```python
from build123d import *

# Parameters (mm, degrees)
EXTRUDE1_DEPTH     = 12.7
SKETCH4_R          = 6.35
CUT_EXTRUDE1_DEPTH = 13.7
CHAMFER2_SIZE      = 0.762


with BuildPart() as part:
    # Sketch2 → Extrude1 (new body)
    with BuildSketch(Plane.XY):
        Polygon((8.798818102, 0), (4.399409051, 7.62), (-4.399409051, 7.62), (-8.798818102, 0), (-4.399409051, -7.62), (4.399409051, -7.62), align=None)
    extrude(amount=EXTRUDE1_DEPTH)

    # Sketch4 → Cut-Extrude1 (cut, through all)
    with BuildSketch(Plane.XY.offset(12.7)):
        Circle(SKETCH4_R)
    extrude(amount=-CUT_EXTRUDE1_DEPTH, mode=Mode.SUBTRACT)

    # Chamfer2
    chamfer2_edges = [part.edges().sort_by_distance(p)[0] for p in [
        (0, 7.62, 12.7),
        (-6.599113577, 3.81, 12.7),
        (-6.599113577, -3.81, 12.7),
        (0, -7.62, 12.7),
        (6.599113577, -3.81, 12.7),
        (6.599113577, 3.81, 12.7),
    ]]
    chamfer(chamfer2_edges, length=CHAMFER2_SIZE)


solid = part.part
```
Check sheet for the modelled part. Datum: model origin and axes. Units: mm. Give positions to 0.01 mm unless a question says otherwise; leave off trailing zeros. Write each loop counter-clockwise with the first axis right and the second up, starting at its lowest first coordinate (ties: lowest second). Pieces come first, ordered by that corner, then holes. Notation, with made-up numbers: (33, 25.5) - (91, 25.5) arc R22 ccw to (91, 64.5) - close; hole circle Ø6 at (82.5, 38). An arc over 180 degrees is marked (long way). Answer as a JSON object with one key per item and string values. Group by question number.
1) Sectioned sample at A-A (x = 0). Record the cut outline in (y, z).
2) Thickness scan on probe 1 along Y at (x, z) = (0, 4.75); probe 2 along Y at (x, z) = (-1.75, 4.5); probe 3 along X at (y, z) = (3.75, 8.5). Record the ranges inside material, lowest first. Write a range as from..to.
3) Release check for a two-part mould opening along X. For faces 1 (the face through (-1.38, -6.2, 6.44)), 2 (the face through (0, -7.62, 6)), 3 (the face through (6.57, -3.86, 5.89)) record: pulls with the +X half, pulls with the -X half, needs draft (parallel to the pull), parting line crosses it, or undercut.
4) Sectioned sample at C-C (z = 10). Record the cut outline in (x, y), then the cut area to 3 significant figures.
5) Depth check by flat-ended pin: P1, Ø3, axis at y = 1, z = 5.5, coming from the +X side; P2, Ø6, axis at y = -5, z = 2.5, coming from the +X side; P3, Ø6, axis at x = 4, y = 4, coming from the +Z side; P4, Ø1.5, axis at y = -3.5, z = 8.5, coming from the -X side. Enter the tip coordinate at first touch or a pass-through.
6) Sectioned sample at B-B (y = -0.75). Record the cut outline in (x, z), then the cut area to 3 significant figures.
Geometry results:
{
 "1": {"outline": "(-7.62, 0) - (-6.35, 0) - (-6.35, 12.7) - (-6.86, 12.7) - (-7.62, 11.94) - close; (6.35, 0) - (7.62, 0) - (7.62, 11.94) - (6.86, 12.7) - (6.35, 12.7) - close"},
 "2": {"probe 1": "y = -7.62..-6.35, 6.35..7.62", "probe 2": "y = -7.62..-6.1, 6.1..7.62", "probe 3": "x = -6.63..-5.12, 5.12..6.63"},
 "3": {"face 1": "undercut", "face 2": "needs draft", "face 3": "pulls with the +X half"},
 "4": {"outline": "(-8.8, 0) - (-4.4, -7.62) - (4.4, -7.62) - (8.8, 0) - (4.4, 7.62) - (-4.4, 7.62) - close; hole circle Ø12.7 at (0, 0)", "area": "74.5 mm^2"},
 "5": {"P1": "stops at x = 8.8", "P2": "stops at x = 7.64", "P3": "stops at z = 12.7", "P4": "stops at x = -7.21"},
 "6": {"outline": "(-8.37, 0) - (-6.31, 0) - (-6.31, 12.7) - (-7.49, 12.7) - (-8.37, 11.94) - close; (6.31, 0) - (8.37, 0) - (8.37, 11.94) - (7.49, 12.7) - (6.31, 12.7) - close", "area": "51.7 mm^2"}
}
